Geometry check sheet. Reference: the model listing, model coordinates, mm. A direction names the side the tool comes from. Round coordinates to 2 decimals unless told otherwise and drop trailing zeros. Order: outer loops, then holes, each group sorted by start corner. A loop starts at its lowest first (then second) coordinate and runs counter-clockwise, first axis right, second up. Notation, with made-up numbers: (1, 40.25) - (53, 40.25) arc R24 cw to (53, 74.25) - close; hole circle Ø2 at (26.5, 43). An arc over 180 degrees is marked (long way). Use a Markdown table: item, result. Add a question column.
(1) Mould release check, pull along Y, two halves, no side actions. Record for faces 1 (the face through (8, -21.35, 149)), 2 (the face through (8, -15, 149)), 3 (the face through (-0.84, -18.22, 209.44)), 4 (the face through (-28.15, -18.94, 94.14)): released by +Y, released by -Y, zero draft, split by the parting line, or undercut.
(2) Section check B-B on x = 25. Record the boundary of the cut face in (y, z), then the cut area to 3 significant figures.
(3) Access from +Z, -Z, +X, -X, +Y, -Y to the whole of each face (thin tool, end or side, straight path). Record for faces 5 (the face through (30, -18, 98.2)), 6 (the face through (-0.96, -18.22, 149.76)).
(4) Gauge pin test, flat ends, axial feed: P1, Ø2, axis at x = 25, z = 105.2, coming from the +Y side; P2, Ø3.5, axis at x = -30, y = -18.175, coming from the -Z side; P3, Ø2, axis at x = 27.5, y = -18.5, coming from the +Z side. Record the tip position at first contact, or that the pin passes through.
(5) Thickness scan on line 1 along X through (y, z) = (-19, 105.2); line 2 along Y through (x, z) = (-30, 96) (3 decimals); line 3 along X through (y, z) = (-19.25, 98). Record the ranges inside material, lowest first. Write a range as [from, to].
(6) Section check A-A on z = 147.45. Record the boundary of the cut face in (x, y).
(7) Section check C-C on x = -30. Record the boundary of the cut face in (y, z) (3 decimals).
(8) Section check D-D on z = 201.5. Record the boundary of the cut face in (x, y).
```python
from build123d import *

# Parameters (mm, degrees)
PARED_B_CHUMACERA_J2_START          = -21.35
CROQUIS1_W                          = 76
CROQUIS1_H                          = 81.25
PARED_B_CHUMACERA_J2_DEPTH          = 6.35
PARED_B_CHUMACERA_J2_REDONDEO_START = -21.35
CROQUIS2_R                          = 38
PARED_B_CHUMACERA_J2_REDONDEO_DEPTH = 6.35
PASO_PERNO_Y_ROSCA_M6_KFL001_START  = -21.35
CROQUIS3_R                          = 6.5
CROQUIS3_R_2                        = 2.5
PASO_PERNO_Y_ROSCA_M6_KFL001_DEPTH  = 6.35
ROSCA_M3_ESCUADRAS_START            = -21.35
CROQUIS4_R                          = 1.25
ROSCA_M3_ESCUADRAS_DEPTH            = 6.35
PASADORES_D4_START                  = 90.2
CROQUIS5_R                          = 2
PASADORES_D4_DEPTH                  = 8
ROSCA_M3_BASES_CINCHO_START         = -21.35
CROQUIS6_R                          = 1.25
ROSCA_M3_BASES_CINCHO_DEPTH         = 6.35
PASO_M3_ESCUADRAS_TUERCA_START      = -21.35
CROQUIS7_R                          = 1.7
PASO_M3_ESCUADRAS_TUERCA_DEPTH      = 6.35
PASO_M3_BASE_CINCHO_TUERCA_START    = -21.35
CROQUIS8_R                          = 1.7
PASO_M3_BASE_CINCHO_TUERCA_DEPTH    = 6.35


with BuildPart() as part:
    # Croquis1 → Pared_B_chumacera_J2 (new body)
    with BuildSketch(Plane(origin=(0, 0, 0), x_dir=(1, 0, 0), z_dir=(0, 1, 0)).offset(PARED_B_CHUMACERA_J2_START)):
        with Locations((0, -130.825)):
            Rectangle(CROQUIS1_W, CROQUIS1_H)
    extrude(amount=PARED_B_CHUMACERA_J2_DEPTH)

    # Croquis2 → Pared_B_chumacera_J2_redondeo (add)
    with BuildSketch(Plane(origin=(0, 0, 0), x_dir=(1, 0, 0), z_dir=(0, 1, 0)).offset(PARED_B_CHUMACERA_J2_REDONDEO_START)):
        with Locations((0, -171.45)):
            Circle(CROQUIS2_R)
    extrude(amount=PARED_B_CHUMACERA_J2_REDONDEO_DEPTH)

    # Croquis3 → Paso_perno_y_rosca_M6_KFL001 (cut)
    with BuildSketch(Plane(origin=(0, 0, 0), x_dir=(1, 0, 0), z_dir=(0, 1, 0)).offset(PASO_PERNO_Y_ROSCA_M6_KFL001_START)):
        with Locations(Location((0, -171.45, 0), (0, 0, 270))):
            Circle(CROQUIS3_R)
        with Locations(Location((0, -195.45, 0), (0, 0, 270))):
            Circle(CROQUIS3_R_2)
        with Locations(Location((0, -147.45, 0), (0, 0, 270))):
            Circle(CROQUIS3_R_2)
    extrude(amount=PASO_PERNO_Y_ROSCA_M6_KFL001_DEPTH, mode=Mode.SUBTRACT)

    # Croquis4 → Rosca_M3_escuadras (cut)
    with BuildSketch(Plane(origin=(0, 0, 0), x_dir=(1, 0, 0), z_dir=(0, 1, 0)).offset(ROSCA_M3_ESCUADRAS_START)):
        with Locations(Location((-25, -105.2, 0), (0, 0, 270))):
            Circle(CROQUIS4_R)
        with Locations(Location((25, -105.2, 0), (0, 0, 270))):
            Circle(CROQUIS4_R)
    extrude(amount=ROSCA_M3_ESCUADRAS_DEPTH, mode=Mode.SUBTRACT)

    # Croquis5 → Pasadores_D4 (cut)
    with BuildSketch(Plane.XY.offset(PASADORES_D4_START)):
        with Locations((-30, -18.175)):
            Circle(CROQUIS5_R)
        with Locations((30, -18.175)):
            Circle(CROQUIS5_R)
    extrude(amount=PASADORES_D4_DEPTH, mode=Mode.SUBTRACT)

    # Croquis6 → Rosca_M3_bases_cincho (cut)
    with BuildSketch(Plane(origin=(0, 0, 0), x_dir=(1, 0, 0), z_dir=(0, 1, 0)).offset(ROSCA_M3_BASES_CINCHO_START)):
        with Locations(Location((0, -117, 0), (0, 0, 270))):
            Circle(CROQUIS6_R)
    extrude(amount=ROSCA_M3_BASES_CINCHO_DEPTH, mode=Mode.SUBTRACT)

    # Croquis7 → Paso_M3_escuadras_tuerca (cut)
    with BuildSketch(Plane(origin=(0, 0, 0), x_dir=(1, 0, 0), z_dir=(0, 1, 0)).offset(PASO_M3_ESCUADRAS_TUERCA_START)):
        with Locations(Location((-25, -105.2, 0), (0, 0, 270))):
            Circle(CROQUIS7_R)
        with Locations(Location((25, -105.2, 0), (0, 0, 270))):
            Circle(CROQUIS7_R)
    extrude(amount=PASO_M3_ESCUADRAS_TUERCA_DEPTH, mode=Mode.SUBTRACT)

    # Croquis8 → Paso_M3_base_cincho_tuerca (cut)
    with BuildSketch(Plane(origin=(0, 0, 0), x_dir=(1, 0, 0), z_dir=(0, 1, 0)).offset(PASO_M3_BASE_CINCHO_TUERCA_START)):
        with Locations(Location((0, -117, 0), (0, 0, 270))):
            Circle(CROQUIS8_R)
    extrude(amount=PASO_M3_BASE_CINCHO_TUERCA_DEPTH, mode=Mode.SUBTRACT)


solid = part.part
```
Check sheet entries:
| question | item | result |
|---|---|---|
| 1 | face 1 | released by -Y |
| 1 | face 2 | released by +Y |
| 1 | face 3 | zero draft |
| 1 | face 4 | undercut |
| 2 | outline | (-21.35, 90.2) - (-15, 90.2) - (-15, 103.5) - (-21.35, 103.5) - close; (-21.35, 106.9) - (-15, 106.9) - (-15, 200.07) - (-21.35, 200.07) - close |
| 2 | area | 676 mm2 |
| 3 | face 5 | -Z |
| 3 | face 6 | +Y, -Y |
| 4 | P1 | passes through |
| 4 | P2 | stops at z = 98.2 |
| 4 | P3 | stops at z = 198.69 |
| 5 | line 1 | x = [-38, -26.7], [-23.3, 23.3], [26.7, 38] |
| 5 | line 2 | y = [-21.35, -20.175], [-16.175, -15] |
| 5 | line 3 | x = [-38, -31.69], [-28.31, 28.31], [31.69, 38] |
| 6 | outline | (-38, -21.35) - (-2.5, -21.35) - (-2.5, -15) - (-38, -15) - close; (2.5, -21.35) - (38, -21.35) - (38, -15) - (2.5, -15) - close |
| 7 | outline | (-21.35, 90.2) - (-20.175, 90.2) - (-20.175, 98.2) - (-16.175, 98.2) - (-16.175, 90.2) - (-15, 90.2) - (-15, 194.774) - (-21.35, 194.774) - close |
| 8 | outline | (-23.26, -21.35) - (23.26, -21.35) - (23.26, -15) - (-23.26, -15) - close |
